For this review, take the finished solid that the model builds, in its own axes (mm). A direction names the side the tool comes from. Give positions to 0.01 mm unless a question says otherwise; leave off trailing zeros. Order: outer loops, then holes, each group sorted by start corner. A loop starts at its lowest first (then second) coordinate and runs counter-clockwise, first axis right, second up. Notation, with made-up numbers: M -36,24.25 L -20,24.25 A23 cw -20,61.25 Z; hole C -4.75,-16.75 d10. An arc over 180 degrees is marked long. Answer as CSV lines item,"result". Start each with the question number.
1. We need section C-C, the plane y = 3.25. Give the boundary of the cut face in (x, z) (3 decimals), and give its area (3 significant figures).
2. We need section D-D, the plane x = -2. Give the boundary of the cut face in (y, z), and give its area (3 significant figures).
3. For line 1 along X through (y, z) = (6, 0) (3 decimals); line 2 along Y through (x, z) = (-5, 0.5); line 3 along Y through (x, z) = (1, 3.5), list the stretches that pass through material, from the lowest coordinate up.
4. Mouldability with a two-part tool opening along Z and no side actions: class faces 4 (the flat face through (3.44, 22.54, -0.1)), 5 (the cylindrical face through (-0.07, 19.29, -0.05)), 6 (the cylindrical face through (-1.93, 9.46, -2.52)) as pulls with the +Z half, pulls with the -Z half, needs draft (parallel to the pull), parting line crosses it, or undercut.
5. We need section A-A, the plane x = 0. Give the boundary of the cut face in (y, z) (3 decimals), and give its area (3 significant figures).
6. Machinability: for faces 1 (the flat face through (0, 21, -3.302)), 2 (the cylindrical face through (-0.345, 4.93, -0.831)), 3 (the flat face through (-1, 0, 1)), which of the approach directions +Z, -Z, +X, -X, +Y, -Y give a long, thin tool a straight path to every point of the face, cutting with its end or side? Answer none if there is none.
7. We need section B-B, the plane z = 0. Give the boundary of the cut face in (x, y) (3 decimals).
8. Clearance check with flat-ended pins moving along their axes: P1, Ø3, axis at x = 2, y = 19.5, coming from the +Z side; P2, Ø3, axis at x = 6, y = 12.5, coming from the +Z side; P3, Ø8, axis at x = -3.5, y = 8, coming from the -Z side (3 decimals); P4, Ø2.5, axis at x = 0, z = 0, coming from the +Y side. State where each tip first meets the part, or that it passes through.
from build123d import *

# Parameters (mm, degrees)
SKETCH1_R               = 3.175
BOSS_EXTRUDE1_DEPTH     = 20
SKETCH2_R               = 0.9
CUT_EXTRUDE1_DEPTH      = 10
SKETCH4_R               = 7.5
BOSS_EXTRUDE2_DEPTH     = 2.54
SKETCH6_R               = 4.85
BOSS_EXTRUDE3_DEPTH     = 3.35
CUT_EXTRUDE3_DEPTH      = 3.3
CUT_EXTRUDE3_DEPTH_BACK = 3.302
SKETCH5_R               = 3.25


with BuildPart() as part:
    # Sketch1 → Boss-Extrude1 (new body)
    with BuildSketch(Plane(origin=(0, 0, 0), x_dir=(1, 0, 0), z_dir=(0, 1, 0))):
        with Locations(Location((0, 0, 0), (0, 0, 270))):
            Circle(SKETCH1_R)
    extrude(amount=BOSS_EXTRUDE1_DEPTH)

    # Sketch2 → Cut-Extrude1 (cut)
    with BuildSketch(Plane.XZ):
        with Locations(Location((0, 0, 0), (0, 0, 270))):
            Circle(SKETCH2_R)
    extrude(amount=-CUT_EXTRUDE1_DEPTH, mode=Mode.SUBTRACT)

    # Sketch4 → Boss-Extrude2 (add)
    with BuildSketch(Plane(origin=(0, 20, 0), x_dir=(1, 0, 0), z_dir=(0, 1, 0))):
        with Locations(Location((0, 0, 0), (0, 0, 270))):
            Circle(SKETCH4_R)
    extrude(amount=BOSS_EXTRUDE2_DEPTH)

    # Sketch6 → Boss-Extrude3 (add)
    with BuildSketch(Plane(origin=(0, 22.54, 0), x_dir=(1, 0, 0), z_dir=(0, 1, 0))):
        with Locations(Location((0, 0, 0), (0, 0, 270))):
            Circle(SKETCH6_R)
    extrude(amount=-BOSS_EXTRUDE3_DEPTH)

    # Sketch5 → Cut-Extrude3 (cut, two sides: drawn at the far end of the back side and taken through both)
    with BuildSketch(Plane.XY.offset(-CUT_EXTRUDE3_DEPTH_BACK)):
        with Locations((0, 22.54)):
            Circle(SKETCH5_R)
    extrude(amount=CUT_EXTRUDE3_DEPTH + CUT_EXTRUDE3_DEPTH_BACK, mode=Mode.SUBTRACT)


solid = part.part
Result set:
1,outline,"C 0,0 d6.35; hole C 0,0 d1.8"
1,area,"29.1 mm2"
2,outline,"M 0,-2.47 L 19.19,-2.47 L 19.19,-4.42 L 20,-4.42 L 20,-7.23 L 22.54,-7.23 L 22.54,-3.3 L 19.98,-3.3 L 19.98,3.3 L 22.54,3.3 L 22.54,7.23 L 20,7.23 L 20,4.42 L 19.19,4.42 L 19.19,2.47 L 0,2.47 Z"
2,area,"122 mm2"
3,line 1,"-3.175 to -0.9, 0.9 to 3.175"
3,line 2,"20 to 22.54"
3,line 3,"19.19 to 22.54"
4,face 4,"needs draft"
4,face 5,"undercut"
4,face 6,"parting line crosses it"
5,outline,"M 0,-3.175 L 19.19,-3.175 L 19.19,-4.85 L 20,-4.85 L 20,-7.5 L 22.54,-7.5 L 22.54,-3.302 L 19.29,-3.302 L 19.29,3.3 L 22.54,3.3 L 22.54,7.5 L 20,7.5 L 20,4.85 L 19.19,4.85 L 19.19,3.175 L 0,3.175 L 0,0.9 L 10,0.9 L 10,-0.9 L 0,-0.9 Z"
5,area,"128 mm2"
6,face 1,"+Y"
6,face 2,"-Y"
6,face 3,"+Z, -Z, +X, -X, -Y"
7,outline,"M -7.5,20 L -4.85,20 L -4.85,19.19 L -3.175,19.19 L -3.175,0 L -0.9,0 L -0.9,10 L 0.9,10 L 0.9,0 L 3.175,0 L 3.175,19.19 L 4.85,19.19 L 4.85,20 L 7.5,20 L 7.5,22.54 L 3.25,22.54 A3.25 cw -3.25,22.54 L -7.5,22.54 Z"
8,P1,"z = 7.48"
8,P2,"through"
8,P3,"z = -3.175"
8,P4,"y = 19.54"
